Answer from the drawing. Dimensions are ordinates in mm from the lowest x, y and z of the part. Give positions to 0.01 mm unless a question says otherwise; leave off trailing zeros. Order: outer loops, then holes, each group sorted by start corner. A loop starts at its lowest first (then second) coordinate and runs counter-clockwise, first axis right, second up.
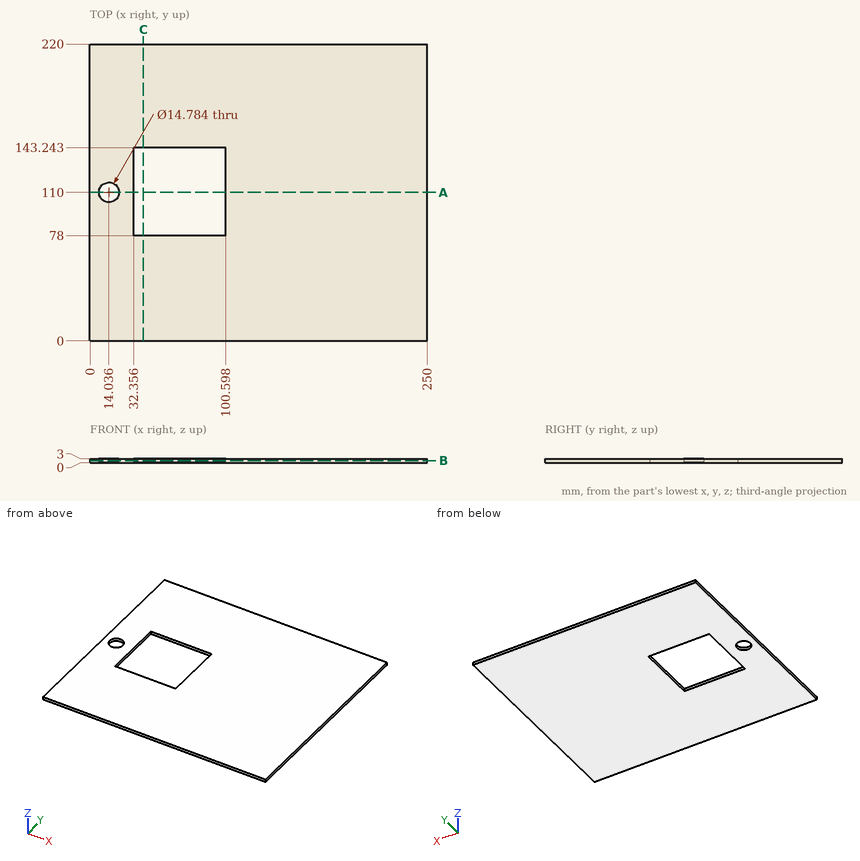
1. The part is cut by section B-B (z = 1.6). Write down the section's boundary in (x, y) (1 decimal).
Findings below:
outline: (0, 0) - (250, 0) - (250, 220) - (0, 220) - close; hole circle Ø14.8 at (14, 110); hole (32.4, 78) - (100.6, 78) - (100.6, 143.2) - (32.4, 143.2) - close
2. The part is cut by section A-A (y = 110). Write down the section's boundary in (x, z) (1 decimal).
Findings below:
outline: (0, 0) - (6.6, 0) - (6.6, 3) - (0, 3) - close; (21.4, 0) - (32.4, 0) - (32.4, 3) - (21.4, 3) - close; (100.6, 0) - (250, 0) - (250, 3) - (100.6, 3) - close
3. The part is cut by section C-C (x = 39.5). Write down the section's boundary in (y, z).
Findings below:
outline: (0, 0) - (78, 0) - (78, 3) - (0, 3) - close; (143.24, 0) - (220, 0) - (220, 3) - (143.24, 3) - close
4. Straight lines are drawn through the part: probe 1 along Y at (x, z) = (92, 2.65); probe 2 along X at (y, z) = (84, 1.7) (1 decimal); probe 3 along X at (y, z) = (113, 2.1) (1 decimal). For each, find the intervals that lie inside material, in ascending order.
Findings below:
probe 1: y = 0 to 78, 143.24 to 220
probe 2: x = 0 to 32.4, 100.6 to 250
probe 3: x = 0 to 7.3, 20.8 to 32.4, 100.6 to 250
